from build123d import *

# Parameters (mm, degrees)
F0_W     = 990.6
F0_H     = 990.6
F1_DEPTH = 152.4
F2_W     = 990.6
F2_H     = 279.4
F3_DEPTH = 152.4
F4_W     = 179.104452
F4_H     = 990.6
F4_W_2   = 227.295548
F5_DEPTH = 152.4


with BuildPart() as f1:
    # F0 (on Top) → F1 (new body)
    with BuildSketch(Plane.XY):
        Rectangle(F0_W, F0_H)
    extrude(amount=F1_DEPTH)

    # F2 (on face) → F3 (join)
    with BuildSketch(Plane.XY.offset(152.4)):
        with Locations((0, 355.6)):
            Rectangle(F2_W, F2_H)
        with Locations((0, -355.6)):
            Rectangle(F2_W, F2_H)
    extrude(amount=F3_DEPTH)

    # F4 (on face) → F5 (join)
    with BuildSketch(Plane(origin=(0, 0, 0), x_dir=(1, 0, 0), z_dir=(0, 0, -1))):
        with Locations((-405.747774, 0)):
            Rectangle(F4_W, F4_H)
        with Locations((381.652226, 0)):
            Rectangle(F4_W_2, F4_H)
    extrude(amount=F5_DEPTH)


solid = f1.part
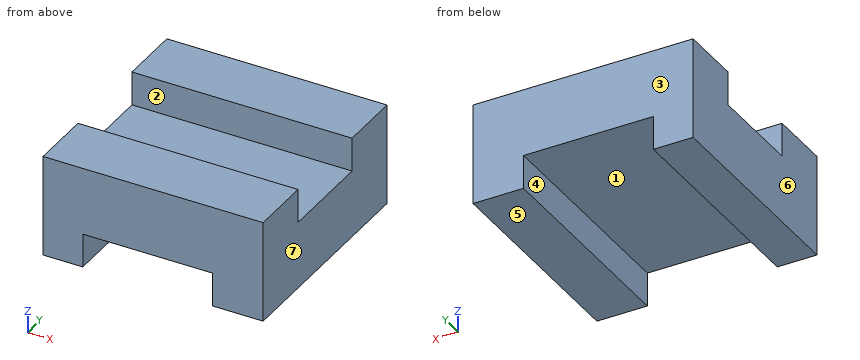
Geometry: final body of the model. Coordinates: model frame, mm. Face numbers are marked on the shaded views. A direction names the side the tool comes from. Coordinates: 2 decimals unless noted, no trailing zeros. Order: outer loops, then holes, each group sorted by start corner. A loop starts at its lowest first (then second) coordinate and runs counter-clockwise, first axis right, second up.
1) Draft query along X for the marked faces 4, 5, 6 and 7. Return one class per face: released by +X, released by -X, zero draft, split by the parting line, or undercut.
Result sheet:
face 4: undercut
face 5: zero draft
face 6: released by -X
face 7: released by +X
2) Set-up query: the marked faces 1, 2 and 3. Return all of +Z, -Z, +X, -X, +Y, -Y with unobstructed straight access to the full face (end or side cutting, diameter ignored); none if empty.
Result sheet:
face 1: -Z, +Y, -Y
face 2: +Z, +X, -X
face 3: +Z, -Z, +X, -X, +Y
3) Section C-C (y = -256.5). Return loops of the section in (x, z), then the cut area to 3 significant figures.
Result sheet:
outline: (-495.3, -152.4) - (-316.2, -152.4) - (-316.2, 0) - (268, 0) - (268, -152.4) - (495.3, -152.4) - (495.3, 304.8) - (-495.3, 304.8) - close
area: 364,000 mm2
4) Section D-D (z = 272). Return loops of the section in (x, y), then the cut area to 3 significant figures.
Result sheet:
outline: (-495.3, -495.3) - (495.3, -495.3) - (495.3, -215.9) - (-495.3, -215.9) - close; (-495.3, 215.9) - (495.3, 215.9) - (495.3, 495.3) - (-495.3, 495.3) - close
area: 554,000 mm2
5) Section B-B (x = 34). Return loops of the section in (y, z), then the cut area to 3 significant figures.
Result sheet:
outline: (-495.3, 0) - (495.3, 0) - (495.3, 304.8) - (215.9, 304.8) - (215.9, 152.4) - (-215.9, 152.4) - (-215.9, 304.8) - (-495.3, 304.8) - close
area: 236,000 mm2
6) Section A-A (z = -69). Return loops of the section in (x, y).
Result sheet:
outline: (-495.3, -495.3) - (-316.2, -495.3) - (-316.2, 495.3) - (-495.3, 495.3) - close; (268, -495.3) - (495.3, -495.3) - (495.3, 495.3) - (268, 495.3) - close
7) Ray query, probe 1 along X at (y, z) = (-174.5, -14.5); probe 2 along Y at (x, z) = (289.5, 216); probe 3 along Z at (x, y) = (-147.5, 136). Return the intervals inside material, ascending.
Result sheet:
probe 1: x = -495.3 to -316.2, 268 to 495.3
probe 2: y = -495.3 to -215.9, 215.9 to 495.3
probe 3: z = 0 to 152.4
